from build123d import *

# Parameters (mm, degrees)
SKETCH1_W           = 249.6
SKETCH1_H           = 267.4
SKETCH1_R           = 2.5
SKETCH1_W_2         = 33
SKETCH1_H_2         = 90
BOSS_EXTRUDE1_DEPTH = 5
CUT_EXTRUDE4_DEPTH  = 6
SKETCH7_W           = 5
SKETCH7_H           = 20
SKETCH7_H_2         = 25
CUT_EXTRUDE5_DEPTH  = 6


with BuildPart() as part:
    # Sketch1 → Boss-Extrude1 (new body)
    with BuildSketch(Plane.XY):
        with Locations((124.8, -202.7)):
            Rectangle(SKETCH1_W, SKETCH1_H)
        with Locations((245.6, -95.5)):
            Circle(SKETCH1_R, mode=Mode.SUBTRACT)
        with Locations((245.6, -146.5)):
            Circle(SKETCH1_R, mode=Mode.SUBTRACT)
        with Locations((4, -146.5)):
            Circle(SKETCH1_R, mode=Mode.SUBTRACT)
        with Locations((4, -95.5)):
            Circle(SKETCH1_R, mode=Mode.SUBTRACT)
        with Locations((201.66, -121)):
            Rectangle(SKETCH1_W_2, SKETCH1_H_2, mode=Mode.SUBTRACT)
        with Locations((47.94, -121)):
            Rectangle(SKETCH1_W_2, SKETCH1_H_2, mode=Mode.SUBTRACT)
    extrude(amount=BOSS_EXTRUDE1_DEPTH)

    # Sketch6 → Cut-Extrude4 (cut, through all)
    with BuildSketch(Plane.XY.offset(5)):
        Polygon((132, -295.148008477), (249.6, -295.148008477), (249.6, -336.4), (0, -336.4), (0, -227), (0, -164), (132, -164), align=None)
        with BuildLine():
            Line((234.205987928, -292), (296.705987928, -292))
            Line((296.705987928, -292), (296.705987928, -167))
            Line((296.705987928, -167), (234.205987928, -167))
            ThreePointArc((234.205987928, -167), (171.705987928, -229.5), (234.205987928, -292))
        make_face()
    extrude(amount=-CUT_EXTRUDE4_DEPTH, mode=Mode.SUBTRACT)

    # Sketch7 → Cut-Extrude5 (cut, through all)
    with BuildSketch(Plane.XY.offset(5)):
        with Locations((15.72, -30.8123203)):
            Rectangle(SKETCH7_W, SKETCH7_H)
        with Locations((233.88, -30.8123203)):
            Rectangle(SKETCH7_W, SKETCH7_H)
        with Locations((15.72, -73.3123203)):
            Rectangle(SKETCH7_W, SKETCH7_H_2)
        with Locations((233.88, -73.3123203)):
            Rectangle(SKETCH7_W, SKETCH7_H_2)
    extrude(amount=-CUT_EXTRUDE5_DEPTH, mode=Mode.SUBTRACT)


solid = part.part
Part model, mm, in its own coordinate system. Coordinates: 2 decimals unless noted, no trailing zeros. Order: outer loops, then holes, each group sorted by start corner. A loop starts at its lowest first (then second) coordinate and runs counter-clockwise, first axis right, second up. Notation, with made-up numbers: M -35.75,48 L -24.75,48 A19 cw -24.75,58 Z; hole C -1.75,13 d9. An arc over 180 degrees is marked long. Use a Markdown table: item, result.
(1) Pull direction Y, two halves, no side cores. Call faces 1 (the cylindrical face through (171.72, -228.13, 2.54)), 2 (the flat face through (123, -130, 0)): released by +Y, released by -Y, zero draft, split by the parting line, or undercut.
A:
| item | result |
|---|---|
| face 1 | undercut |
| face 2 | zero draft |
(2) Flat gauge pins, fed straight in: pin 1 (2.5 mm diameter, centred on y = -207, z = 2.5, fed in from -X); pin 2 (6 mm diameter, centred on x = 245.6, y = -95.5, fed in from +Z); pin 3 (1 mm diameter, centred on x = 53.5, z = 2.5, fed in from -Y); pin 4 (1.5 mm diameter, centred on x = 233, z = 3.5, fed in from +Y). Where does each tip first touch, or does it go through?
A:
| item | result |
|---|---|
| pin 1 | stops at x = 132 |
| pin 2 | stops at z = 5 |
| pin 3 | stops at y = -76 |
| pin 4 | stops at y = -85.81 |
(3) Cut at C-C on x = 49.5. Write the cut outline in (y, z), then the cut area to 3 significant figures.
A:
| item | result |
|---|---|
| outline | M -76,0 L -69,0 L -69,5 L -76,5 Z |
| area | 35.0 mm^2 |
(4) Cut at A-A on y = -156.5. Write the cut outline in (x, z), then the cut area to 3 significant figures.
A:
| item | result |
|---|---|
| outline | M 0,0 L 31.44,0 L 31.44,5 L 0,5 Z; M 64.44,0 L 185.16,0 L 185.16,5 L 64.44,5 Z; M 218.16,0 L 249.6,0 L 249.6,5 L 218.16,5 Z |
| area | 918 mm^2 |
(5) Cut at D-D on y = -229.5. Write the cut outline in (x, z), then the cut area to 3 significant figures.
A:
| item | result |
|---|---|
| outline | M 132,0 L 171.71,0 L 171.71,5 L 132,5 Z |
| area | 199 mm^2 |
(6) Probe L1, parallel to X at y = -146.5, z = 3.3; L2, parallel to Y at x = 245.6, z = 3.9; L3, parallel to X at y = -153.5, z = 2.55. List the from-to ranges inside material, lowest first.
A:
| item | result |
|---|---|
| L1 | x = 0 to 1.5, 6.5 to 31.44, 64.44 to 185.16, 218.16 to 243.1, 248.1 to 249.6 |
| L2 | y = -295.15 to -292, -167 to -149, -144 to -98, -93 to -69 |
| L3 | x = 0 to 31.44, 64.44 to 185.16, 218.16 to 249.6 |
(7) Cut at B-B on z = 0.8. State how many separate pieces and enclosed holes the cut face has, then the cut area to 3 significant figures.
A:
| item | result |
|---|---|
| separate pieces | 1 |
| enclosed holes | 5 |
| area | 25,000 mm^2 |
